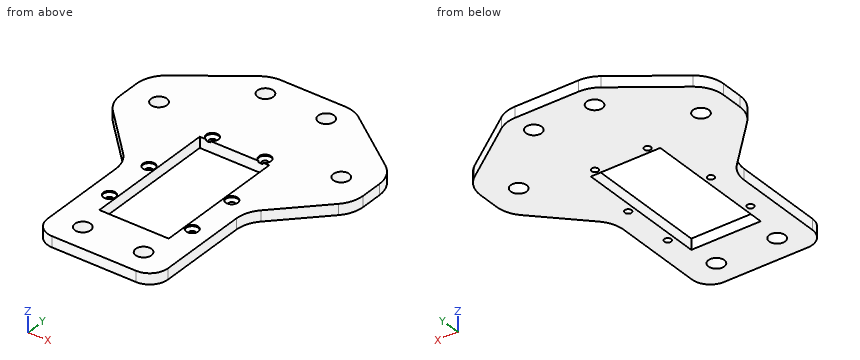
```python
from build123d import *

# Parameters (mm, degrees)
F0_R         = 3.302
F0_R_2       = 1.397
F1_DEPTH     = 4.4958
F3_R         = 2.54
F4_DEPTH     = 0.381
F5_S5_R      = 2.54
F5_T6_DEPTH  = 5
F5_S11_R     = 2.54
F5_T12_DEPTH = 5
F5_S17_R     = 2.54
F5_T18_DEPTH = 5
F5_S23_R     = 2.54
F5_T24_DEPTH = 5
F5_S29_R     = 2.54
F5_T30_DEPTH = 5
F5_S35_R     = 2.54
F5_T36_DEPTH = 5


# Not quite as in the source:
# - a fillet or chamfer that OpenCascade refuses, or shapes differently, is made with other operations: its cross-section is extruded or revolved along the edge and cut away or added


with BuildPart() as f1:
    # F0 (on Top) → F1 (new body)
    with BuildSketch(Plane.XY):
        with BuildLine():
            Line((0, 71.7569190334), (-13.3202167361, 71.7569190334))
            ThreePointArc((-13.3202167361, 71.7569190334), (-17.2583195593, 71.1309136563), (-20.8081903285, 69.3146113411))
            Line((-20.8081903285, 69.3146113411), (-45.5879735924, 51.2257120897))
            ThreePointArc((-45.5879735924, 51.2257120897), (-49.4222626852, 46.7209640446), (-50.8, 40.968019782))
            Line((-50.8, 40.968019782), (-50.8, 31.9697443563))
            ThreePointArc((-50.8, 31.9697443563), (-49.8574337411, 27.1684162251), (-47.1696453822, 23.0797762663))
            Line((-47.1696453822, 23.0797762663), (-28.8017546178, 4.3406476252))
            ThreePointArc((-28.8017546178, 4.3406476252), (-26.1139662589, 0.2520076664), (-25.1714, -4.5493204647))
            Line((-25.1714, -4.5493204647), (-25.1714, -42.5430809666))
            ThreePointArc((-25.1714, -42.5430809666), (-22.9395536726, -47.9312346392), (-17.5514, -50.1630809666))
            Line((-17.5514, -50.1630809666), (0, -50.1630809666))
            Line((0, -50.1630809666), (0, -27.9380809666))
            Line((0, -27.9380809666), (-14.5034, -27.9380809666))
            Line((-14.5034, -27.9380809666), (-14.5034, 27.9419190334))
            Line((-14.5034, 27.9419190334), (0, 27.9419190334))
            Line((0, 27.9419190334), (0, 71.7569190334))
        make_face()
        with Locations((-12.7, -39.5204809666)):
            Circle(F0_R, mode=Mode.SUBTRACT)
        with Locations((-17.2974, -18.5654809666)):
            Circle(F0_R_2, mode=Mode.SUBTRACT)
        with Locations((-17.2974, 3.4309190334)):
            Circle(F0_R_2, mode=Mode.SUBTRACT)
        with Locations((-38.1, 36.6795190334)):
            Circle(F0_R, mode=Mode.SUBTRACT)
        with Locations((-10.9982, 30.3231690334)):
            Circle(F0_R_2, mode=Mode.SUBTRACT)
        with Locations((-12.7, 62.0795190334)):
            Circle(F0_R, mode=Mode.SUBTRACT)
    extrude(amount=F1_DEPTH)

    # F2: F1 across face


with BuildPart() as f1_1:
    add(f1.part)
    add(f1.part.mirror(Plane(origin=(0, 49.8494190334, 2.2479), x_dir=(0, 1, 0), z_dir=(1, 0, 0))))

    # F3 (on face) → F4 (cut)
    with BuildSketch(Plane.XY.offset(4.4958)):
        with Locations((-10.9982, 30.3231690334)):
            Circle(F3_R)
        with Locations((-17.2974, 3.4309190334)):
            Circle(F3_R)
        with Locations((-17.2974, -18.5654809666)):
            Circle(F3_R)
        with Locations((10.9982, 30.3231690334)):
            Circle(F3_R)
        with Locations((17.2974, 3.4309190334)):
            Circle(F3_R)
        with Locations((17.2974, -18.5654809666)):
            Circle(F3_R)
    extrude(amount=-F4_DEPTH, mode=Mode.SUBTRACT)

    # F5: chamfer of 1.27 on 6 edges, made by hand


with BuildPart() as f5_tool2:
    # F5_s3 → F5_t4 (revolve)
    with BuildSketch(Plane.XZ.offset(-30.3231690334)):
        Polygon((-8.3312, 4.1148), (-9.6012, 2.8448), (-9.6012, 4.1148), align=None)
    revolve(axis=Axis((-10.9982, 30.3231690334, 4.1148), (0, 0, -1)))

    # F5_s5 → F5_t6 (intersect, symmetric)
    with BuildSketch(Plane.XY.offset(3.5)):
        with Locations((-10.9982, 30.3231690334)):
            Circle(F5_S5_R)
    extrude(amount=F5_T6_DEPTH, both=True, mode=Mode.INTERSECT)


with BuildPart() as f1_2:
    add(f1_1.part)

    # F5_t1: cut F5_tool2
    add(f5_tool2.part, mode=Mode.SUBTRACT)


with BuildPart() as f5_tool8:
    # F5_s9 → F5_t10 (revolve)
    with BuildSketch(Plane.XZ.offset(-30.3231690334)):
        Polygon((8.3312, 4.1148), (9.6012, 2.8448), (9.6012, 4.1148), align=None)
    revolve(axis=Axis((10.9982, 30.3231690334, 4.1148), (0, 0, -1)))

    # F5_s11 → F5_t12 (intersect, symmetric)
    with BuildSketch(Plane.XY.offset(3.5)):
        with Locations((10.9982, 30.3231690334)):
            Circle(F5_S11_R)
    extrude(amount=F5_T12_DEPTH, both=True, mode=Mode.INTERSECT)


with BuildPart() as f1_3:
    add(f1_2.part)

    # F5_t7: cut F5_tool8
    add(f5_tool8.part, mode=Mode.SUBTRACT)


with BuildPart() as f5_tool14:
    # F5_s15 → F5_t16 (revolve)
    with BuildSketch(Plane.XZ.offset(-3.4309190334)):
        Polygon((-14.6304, 4.1148), (-15.9004, 2.8448), (-15.9004, 4.1148), align=None)
    revolve(axis=Axis((-17.2974, 3.4309190334, 4.1148), (0, 0, -1)))

    # F5_s17 → F5_t18 (intersect, symmetric)
    with BuildSketch(Plane.XY.offset(3.5)):
        with Locations((-17.2974, 3.4309190334)):
            Circle(F5_S17_R)
    extrude(amount=F5_T18_DEPTH, both=True, mode=Mode.INTERSECT)


with BuildPart() as f1_4:
    add(f1_3.part)

    # F5_t13: cut F5_tool14
    add(f5_tool14.part, mode=Mode.SUBTRACT)


with BuildPart() as f5_tool20:
    # F5_s21 → F5_t22 (revolve)
    with BuildSketch(Plane.XZ.offset(-3.4309190334)):
        Polygon((14.6304, 4.1148), (15.9004, 2.8448), (15.9004, 4.1148), align=None)
    revolve(axis=Axis((17.2974, 3.4309190334, 4.1148), (0, 0, -1)))

    # F5_s23 → F5_t24 (intersect, symmetric)
    with BuildSketch(Plane.XY.offset(3.5)):
        with Locations((17.2974, 3.4309190334)):
            Circle(F5_S23_R)
    extrude(amount=F5_T24_DEPTH, both=True, mode=Mode.INTERSECT)


with BuildPart() as f1_5:
    add(f1_4.part)

    # F5_t19: cut F5_tool20
    add(f5_tool20.part, mode=Mode.SUBTRACT)


with BuildPart() as f5_tool26:
    # F5_s27 → F5_t28 (revolve)
    with BuildSketch(Plane.XZ.offset(18.5654809666)):
        Polygon((-14.6304, 4.1148), (-15.9004, 2.8448), (-15.9004, 4.1148), align=None)
    revolve(axis=Axis((-17.2974, -18.5654809666, 4.1148), (0, 0, -1)))

    # F5_s29 → F5_t30 (intersect, symmetric)
    with BuildSketch(Plane.XY.offset(3.5)):
        with Locations((-17.2974, -18.5654809666)):
            Circle(F5_S29_R)
    extrude(amount=F5_T30_DEPTH, both=True, mode=Mode.INTERSECT)


with BuildPart() as f1_6:
    add(f1_5.part)

    # F5_t25: cut F5_tool26
    add(f5_tool26.part, mode=Mode.SUBTRACT)


with BuildPart() as f5_tool32:
    # F5_s33 → F5_t34 (revolve)
    with BuildSketch(Plane.XZ.offset(18.5654809666)):
        Polygon((14.6304, 4.1148), (15.9004, 2.8448), (15.9004, 4.1148), align=None)
    revolve(axis=Axis((17.2974, -18.5654809666, 4.1148), (0, 0, -1)))

    # F5_s35 → F5_t36 (intersect, symmetric)
    with BuildSketch(Plane.XY.offset(3.5)):
        with Locations((17.2974, -18.5654809666)):
            Circle(F5_S35_R)
    extrude(amount=F5_T36_DEPTH, both=True, mode=Mode.INTERSECT)


with BuildPart() as f1_7:
    add(f1_6.part)

    # F5_t31: cut F5_tool32
    add(f5_tool32.part, mode=Mode.SUBTRACT)


solid = f1_7.part
```
CAD build for the part. Positions are in the model's coordinates, mm. Coordinates: 2 decimals unless noted, no trailing zeros. Loops run counter-clockwise (first coordinate to the right, second up) from the corner with the lowest first, then second, coordinate; pieces in that order, holes last. Notation, with made-up numbers: (-4, 69) - (36, 69) arc R35 ccw to (36, 106) - close; hole circle Ø1 at (81.5, 4). An arc over 180 degrees is marked (long way). Use CSV: the item, a comma, the result in double quotes. Start each with the question number.
Q1. Cut at C-C, the plane y = 63.5. List the corners of the cut face in (x, z).
Q2. Drop flat-ended pins along their axis: P1, Ø3.5, axis at x = 17.3, y = 3.43, coming from the +Z side; P2, Ø2, axis at y = -32.5, z = 2, coming from the +X side; P3, Ø4, axis at x = -17.3, y = -18.57, coming from the +Z side. Give the stop position or say it passes through.
Q3. Cut at D-D, the plane z = 1.65. State how many separate pieces and enclosed holes the cut face has, then the cut area to 3 significant figures.
Q4. Probe probe 1 along Y at (x, z) = (12.7, 2.7); probe 2 along Y at (x, z) = (-14, 2.55); probe 3 along X at (y, z) = (-7, 1.7). List the from-to ranges inside material, lowest first. Write a range as from..to.
Q5. Cut at B-B, the plane x = 37. List the corners of the cut face in (y, z), then the cut area to 3 significant figures.
Q6. Cut at A-A, the plane y = 20.5. List the corners of the cut face in (x, z).
Here are the results:
1,outline,"(-28.77, 0) - (-15.68, 0) - (-15.68, 4.5) - (-28.77, 4.5) - close; (-9.72, 0) - (9.72, 0) - (9.72, 4.5) - (-9.72, 4.5) - close; (15.68, 0) - (28.77, 0) - (28.77, 4.5) - (15.68, 4.5) - close"
2,P1,"z = 3.2"
2,P2,"x = 25.17"
2,P3,"z = 3.45"
3,separate pieces,"1"
3,enclosed holes,"13"
3,area,"6,400 mm2"
4,probe 1,"-50.16..-42.82, -36.22..-27.94, 27.94..58.78, 65.38..71.76"
4,probe 2,"-50.16..-42.56, -36.49..-27.94, 27.94..59.04, 65.11..71.74"
4,probe 3,"-25.17..-14.5, 14.5..25.17"
5,outline,"(12.7, 0) - (33.57, 0) - (33.57, 4.5) - (12.7, 4.5) - close; (39.79, 0) - (57.49, 0) - (57.49, 4.5) - (39.79, 4.5) - close"
5,area,"173 mm2"
6,outline,"(-44.64, 0) - (-14.5, 0) - (-14.5, 4.5) - (-44.64, 4.5) - close; (14.5, 0) - (44.64, 0) - (44.64, 4.5) - (14.5, 4.5) - close"
